Read the model definition and answer for the solid it produces. Units are mm, in the model's axes. A direction names the side the tool comes from. Coordinates: 2 decimals unless noted, no trailing zeros. Order: outer loops, then holes, each group sorted by start corner. A loop starts at its lowest first (then second) coordinate and runs counter-clockwise, first axis right, second up.
```python
from build123d import *

# Parameters (mm, degrees)
SKETCH3_R           = 3
SKETCH3_R_2         = 2.5
BOSS_EXTRUDE2_DEPTH = 3
FILLET1_R           = 10
CUT_EXTRUDE1_DEPTH  = 10
FILLET2_R           = 3.75


with BuildPart() as part:
    # Sketch3 → Boss-Extrude2 (new body)
    with BuildSketch(Plane(origin=(0, 0, 0), x_dir=(0, 0, -1), z_dir=(1, 0, 0))):
        with BuildLine():
            Line((7.171582169, 19.591665787), (82.171582169, 41.707880218))
            ThreePointArc((82.171582169, 41.707880218), (85.373366716, 42.109241865), (88.536274395, 41.470077986))
            Line((88.536274395, 41.470077986), (147.036274395, 19.353863555))
            ThreePointArc((147.036274395, 19.353863555), (152.853863555, 6.463725605), (139.963725605, 0.646136445))
            Line((139.963725605, 0.646136445), (100.980229255, 15.384040113))
            Line((100.980229255, 15.384040113), (100.980229255, -1.493532665))
            ThreePointArc((100.980229255, -1.493532665), (90.980229255, -11.493532665), (80.980229255, -1.493532665))
            Line((80.980229255, -1.493532665), (80.980229255, 20.505135217))
            Line((80.980229255, 20.505135217), (12.828417831, 0.408334213))
            ThreePointArc((12.828417831, 0.408334213), (0.408334213, 7.171582169), (7.171582169, 19.591665787))
        make_face()
        with Locations((85, 32.116214431)):
            Circle(SKETCH3_R, mode=Mode.SUBTRACT)
        with Locations((90.980229255, -1.493532665)):
            Circle(SKETCH3_R_2, mode=Mode.SUBTRACT)
        with Locations((10, 10)):
            Circle(SKETCH3_R_2, mode=Mode.SUBTRACT)
        with BuildLine():
            Line((146.6, 12.683281573), (146.6, 7.316718427))
            ThreePointArc((146.6, 7.316718427), (139.4, 10), (146.6, 12.683281573))
        make_face(mode=Mode.SUBTRACT)
    extrude(amount=BOSS_EXTRUDE2_DEPTH)

    # Fillet1
    fillet1_edges = [part.edges().sort_by_distance(p)[0] for p in [
        (1.5, 20.505135217, -80.980229255),
        (1.5, 15.384040113, -100.980229255),
    ]]
    fillet(fillet1_edges, radius=FILLET1_R)

    # Sketch5 → Cut-Extrude1 (cut)
    with BuildSketch(Plane(origin=(0, 0, 0), x_dir=(0, 0, -1), z_dir=(1, 0, 0))):
        Polygon((23.326841994, 17.839501416), (61.693505144, 29.153172739), (63.814818517, 21.959423399), (25.448155367, 10.645752076), align=None)
        with BuildLine():
            Line((86.060882319, 34.922373497), (109.445541205, 26.081687509))
            Line((109.445541205, 26.081687509), (90.980229255, 11.910433147))
            Line((90.980229255, 11.910433147), (82.273860108, 30.863951963))
            ThreePointArc((82.273860108, 30.863951963), (82.806608326, 34.162927153), (86.060882319, 34.922373497))
        make_face()
    extrude(amount=CUT_EXTRUDE1_DEPTH, mode=Mode.SUBTRACT)

    # Fillet2
    fillet2_edges = [part.edges().sort_by_distance(p)[0] for p in [
        (1.5, 11.910433147, -90.980229255),
        (1.5, 26.081687509, -109.445541205),
        (1.5, 29.153172739, -61.693505144),
        (1.5, 21.959423399, -63.814818517),
        (1.5, 10.645752076, -25.448155367),
        (1.5, 17.839501416, -23.326841994),
    ]]
    fillet(fillet2_edges, radius=FILLET2_R - 0.0001)  # a hair under: the kernel refuses the full size


solid = part.part
```
1) A cutting plane is placed at B-B, the plane z = -36. Determine the outline of the cut face in (x, y), and give its area (3 significant figures).
A:
outline: (0, 7.24) - (3, 7.24) - (3, 13.76) - (0, 13.76) - close; (0, 21.58) - (3, 21.58) - (3, 28.09) - (0, 28.09) - close
area: 39.1 mm2
2) Which of the six approach directions +Z, -Z, +X, -X, +Y, -Y give full straight-line access (tool end or side, diameter ignored) to faces 5 (the flat face through (1.48, 8.68, -40.88)), 6 (the cylindrical face through (1.52, 27.81, -60.91)), 7 (the flat face through (1.479, 30.495, -44.147))?
A:
face 5: +X, -X, -Y
face 6: +X, -X
face 7: +Z, +X, -X, +Y
3) A cutting plane is placed at A-A, the plane x = 0.85. State how many separate pieces and enclosed holes the cut face has, and give its area (3 significant figures).
A:
separate pieces: 1
enclosed holes: 5
area: 3,110 mm2
4) Flat-ended cylindrical pins translate along their axes: pin 1 Ø1 at (x, y) = (2, 8) entering from -Z; pin 2 Ø1.5 at (x, z) = (1.5, -110.5) entering from +Y; pin 3 Ø8 at (y, z) = (7.5, -53) entering from +X; pin 4 Ø1.5 at (x, y) = (2, 3.5) entering from +Z. Find the tip coordinate at first contact, or state that the pin passes through.
A:
pin 1: stops at z = -153.39
pin 2: stops at y = 33.45
pin 3: passes through
pin 4: stops at z = -1.82
5) A cutting plane is placed at D-D, the plane z = -66. Determine the outline of the cut face in (x, y), and give its area (3 significant figures).
A:
outline: (0, 16.09) - (3, 16.09) - (3, 36.94) - (0, 36.94) - close
area: 62.6 mm2
6) A cutting plane is placed at C-C, the plane y = 33.5. Determine the outline of the cut face in (x, z), and give its area (3 significant figures).
A:
outline: (0, -109.62) - (3, -109.62) - (3, -89.82) - (0, -89.82) - close; (0, -82.34) - (3, -82.34) - (3, -54.34) - (0, -54.34) - close
area: 143 mm2
7) Determine the mould class of faces 1 (the flat face through (1.479, 30.567, -117.377)), 2 (the cylindrical face through (1.48, 34.2, -82.84)), 3 (the cylindrical face through (1.48, 42.11, -85.33)), 4 (the flat face through (0, 15, -83)) for opening direction Z: pulls with the +Z half, pulls with the -Z half, needs draft (parallel to the pull), parting line crosses it, or undercut.
A:
face 1: pulls with the -Z half
face 2: undercut
face 3: parting line crosses it
face 4: needs draft
8) Straight lines are drawn through the part: line 1 (Y direction, x = 1.8, z = -90); line 2 (Y direction, x = 2.2, z = -54); line 3 (Y direction, x = 2.1, z = -142.5). For each, find the intervals that lie inside material, in ascending order.
A:
line 1: y = -11.45 to -3.79, 0.81 to 14.89, 33.43 to 40.92
line 2: y = 12.55 to 19.07, 26.88 to 33.4
line 3: y = 0.05 to 6.02, 13.98 to 21.07
